Can you work these out from the drawing? Everything is in mm from the part's minimum corner. A direction names the side the tool comes from. Coordinates: 2 decimals unless noted, no trailing zeros. Write each loop counter-clockwise with the first axis right and the second up, starting at its lowest first coordinate (ties: lowest second). Pieces come first, ordered by that corner, then holes. Notation, with made-up numbers: (15.25, -24) -> (72.25, -24) arc R21 ccw to (72.25, 8) -> close; hole circle Ø4 at (-25, -15.75). An arc over 180 degrees is marked (long way). Use CSV: the item, a comma, the result in double quotes. Start each with the question number.
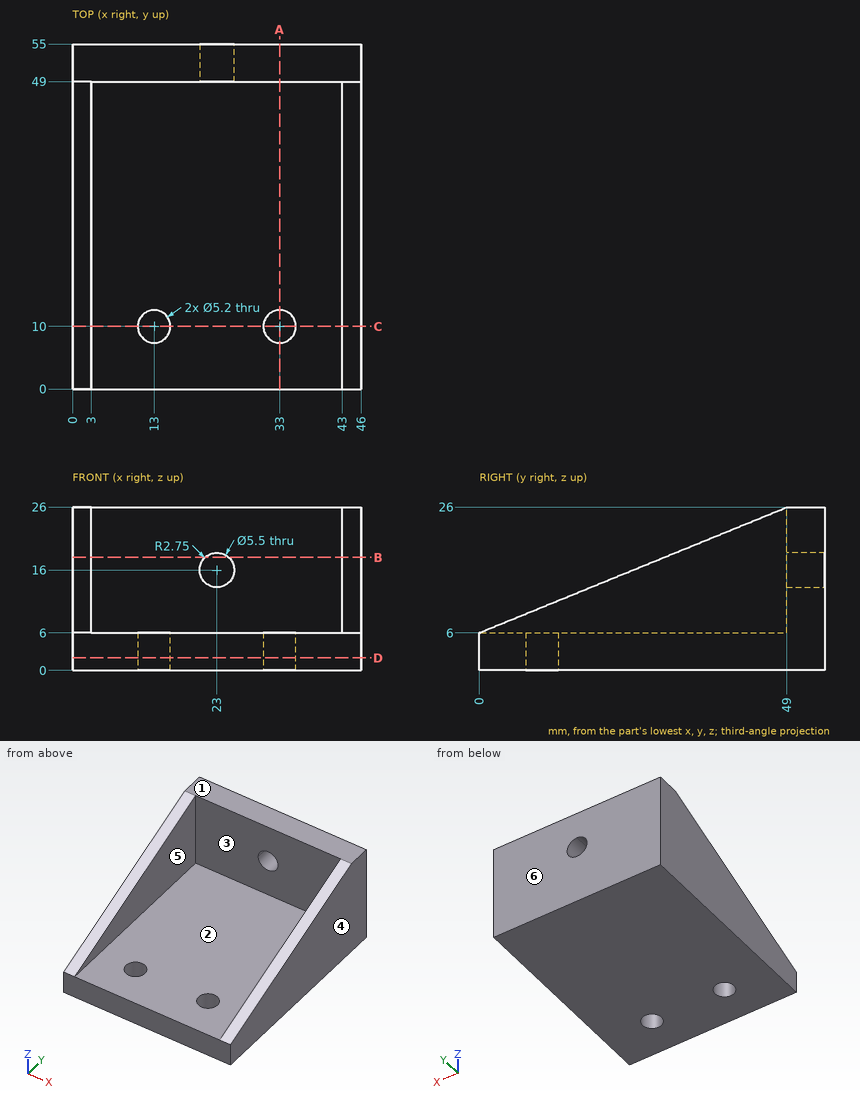
Item 1: I want a section at B-B on z = 18. Please give me the cut outline in (x, y), then the cut area to 3 significant figures.
Item 2: I want a section at C-C on y = 10. Please give me the cut outline in (x, z).
Item 3: I want a section at A-A on x = 33. Please give me the cut outline in (y, z).
Item 4: If I drill on line 1 along Y through (x, z) = (13, 3.1); line 2 along Z through (x, y) = (23, 51.65); line 3 along X through (y, z) = (27, 6.75), over which ranges is the centre line in solid material (lowest first)?
Item 5: I'm going to push flat-ended pins straight in: pin 1 (2 mm diameter, centred on x = 34, z = 20, fed in from -Y); pin 2 (3 mm diameter, centred on x = 33, y = 10, fed in from +Z). Where does each tip first touch, or does it pass through?
Item 6: Thinking about a two-plate mould opening in X: for the marked faces 1, 2, 3 and 4, which applies, +X half, -X half, draft (parallel to the pull), parting line (faces both ways), or undercut?
Item 7: I want a section at D-D on z = 2. Please give me the cut outline in (x, y).
Item 8: Which directions (+Z, -Z, +X, -X, +Y, -Y) give clear straight access to the entire face, cutting with the end or side of a thin tool? Please do the marked faces 5 and 6.
Geometry says:
1,outline,"(0, 29.4) -> (3, 29.4) -> (3, 49) -> (21.11, 49) -> (21.11, 55) -> (0, 55) -> close; (24.89, 49) -> (43, 49) -> (43, 29.4) -> (46, 29.4) -> (46, 55) -> (24.89, 55) -> close"
1,area,"371 mm2"
2,outline,"(0, 0) -> (10.4, 0) -> (10.4, 6) -> (3, 6) -> (3, 10.08) -> (0, 10.08) -> close; (15.6, 0) -> (30.4, 0) -> (30.4, 6) -> (15.6, 6) -> close; (35.6, 0) -> (46, 0) -> (46, 10.08) -> (43, 10.08) -> (43, 6) -> (35.6, 6) -> close"
3,outline,"(0, 0) -> (7.4, 0) -> (7.4, 6) -> (0, 6) -> close; (12.6, 0) -> (55, 0) -> (55, 26) -> (49, 26) -> (49, 6) -> (12.6, 6) -> close"
4,line 1,"0 to 7.4, 12.6 to 55"
4,line 2,"0 to 13.25, 18.75 to 26"
4,line 3,"0 to 3, 43 to 46"
5,pin 1,"y = 49"
5,pin 2,"through"
6,face 1,"draft"
6,face 2,"undercut"
6,face 3,"undercut"
6,face 4,"+X half"
7,outline,"(0, 0) -> (46, 0) -> (46, 55) -> (0, 55) -> close; hole circle Ø5.2 at (13, 10); hole circle Ø5.2 at (33, 10)"
8,face 5,"+Z, -Y"
8,face 6,"+Z, -Z, +X, -X, +Y"
